Part model, mm, in its own coordinate system. A direction names the side the tool comes from. Give positions to 0.01 mm unless a question says otherwise; leave off trailing zeros. Order: outer loops, then holes, each group sorted by start corner. A loop starts at its lowest first (then second) coordinate and runs counter-clockwise, first axis right, second up. Notation, with made-up numbers: (-19, 69.25) - (-12, 69.25) arc R23 cw to (-12, 96.25) - close; hole circle Ø4 at (40, -25.75). An arc over 180 degrees is marked (long way). Use a Markdown table: item, result. Add a question column.
from build123d import *

# Parameters (mm, degrees)
EXTRUDE031_DEPTH = 1
EXTRUDE030_DEPTH = 2.75


with BuildPart() as extrude031:
    # Sketch034 → Extrude031 (new body)
    with BuildSketch(Plane.XZ):
        with BuildLine():
            ThreePointArc((11.7, 16.35), (11.063604, 16.086396), (10.8, 15.45))
            Line((10.8, 14.2), (10.8, 15.45))
            ThreePointArc((10.8, 14.2), (11.23934, 13.13934), (12.3, 12.7))
            Line((16.8, 12.7), (12.3, 12.7))
            ThreePointArc((16.8, 12.7), (17.86066, 13.13934), (18.3, 14.2))
            Line((18.3, 15.45), (18.3, 14.2))
            ThreePointArc((18.3, 15.45), (18.036396, 16.086396), (17.4, 16.35))
            Line((11.7, 16.35), (17.4, 16.35))
        make_face()
    extrude(amount=EXTRUDE031_DEPTH)


with BuildPart() as extrude031_1:
    # Extrude031 placement: moved
    add(extrude031.part.moved(Location((0, 2.5, 0))))


with BuildPart() as button002:
    # Sketch033 → Extrude030 (new body)
    with BuildSketch(Plane.XZ):
        with BuildLine():
            ThreePointArc((12.75, 16.13), (12.113604, 15.866396), (11.85, 15.23))
            Line((11.85, 14.43), (11.85, 15.23))
            ThreePointArc((11.85, 14.43), (12.113604, 13.793604), (12.75, 13.53))
            Line((16.55, 13.53), (12.75, 13.53))
            ThreePointArc((16.55, 13.53), (17.186396, 13.793604), (17.45, 14.43))
            Line((17.45, 15.23), (17.45, 14.43))
            ThreePointArc((17.45, 15.23), (17.186396, 15.866396), (16.55, 16.13))
            Line((12.75, 16.13), (16.55, 16.13))
        make_face()
    extrude(amount=EXTRUDE030_DEPTH)


with BuildPart() as button002_1:
    # Extrude030 placement: moved
    add(button002.part.moved(Location((0, 2, 0))))

    # Fusion033: union Extrude031
    add(extrude031_1.part)


with BuildPart() as button002_2:
    # Fusion033 placement: moved
    add(button002_1.part.moved(Location((32.45, 0, 0))))


solid = button002_2.part
1. Cut at D-D (z = 13.45). Write the cut outline in (x, y).
2. Cut at C-C (x = 50.25). Write the cut outline in (y, z).
3. Cut at A-A (z = 14.8). Write the cut outline in (x, y), plus the area to 3 significant figures.
4. Cut at B-B (y = 1.95). Write the cut outline in (x, z).
5. Pin check, flat tips, straight feed: P1, Ø1.5, axis at y = 1, z = 16, coming from the -X side; P2, Ø0.7, axis at x = 47.5, y = 0.5, coming from the +Z side; P3, Ø0.6, axis at y = 0, z = 14.5, coming from the -X side; P4, Ø0.9, axis at y = 0, z = 15, coming from the +X side. Stop position of each tip, or through.
6. Tool access for faces 1 (the face through (47, 0, 16.13)), 2 (the face through (47, 0, 13.53)), 3 (the face through (47, 1.5, 13)): list every direction of +Z, -Z, +X, -X, +Y, -Y with a clear straight run to the whole face (end or side of a thin tool).
7. Drill centre lines: probe 1 along Z at (x, y) = (47, 0.15); probe 2 along Y at (x, z) = (50, 16.25); probe 3 along X at (y, z) = (1.1, 14.7). Where is each one in solid material? Low to high. Write a range as [from, to].
Responses:
| question | item | result |
|---|---|---|
| 1 | outline | (43.45, 1.5) - (50.55, 1.5) - (50.55, 2.5) - (43.45, 2.5) - close |
| 2 | outline | (1.5, 13.08) - (2.5, 13.08) - (2.5, 16.26) - (1.5, 16.26) - close |
| 3 | outline | (43.25, 1.5) - (44.3, 1.5) - (44.3, -0.75) - (49.9, -0.75) - (49.9, 1.5) - (50.75, 1.5) - (50.75, 2.5) - (43.25, 2.5) - close |
| 3 | area | 20.1 mm² |
| 4 | outline | (43.25, 14.2) arc R1.5 ccw to (44.75, 12.7) - (49.25, 12.7) arc R1.5 ccw to (50.75, 14.2) - (50.75, 15.45) arc R0.9 ccw to (49.85, 16.35) - (44.15, 16.35) arc R0.9 ccw to (43.25, 15.45) - close |
| 5 | P1 | stops at x = 43.25 |
| 5 | P2 | stops at z = 16.13 |
| 5 | P3 | stops at x = 44.3 |
| 5 | P4 | stops at x = 49.9 |
| 6 | face 1 | +Z, +X, -X, -Y |
| 6 | face 2 | -Z, +X, -X, -Y |
| 6 | face 3 | -Y |
| 7 | probe 1 | z = [13.53, 16.13] |
| 7 | probe 2 | y = [1.5, 2.5] |
| 7 | probe 3 | x = [44.3, 49.9] |
